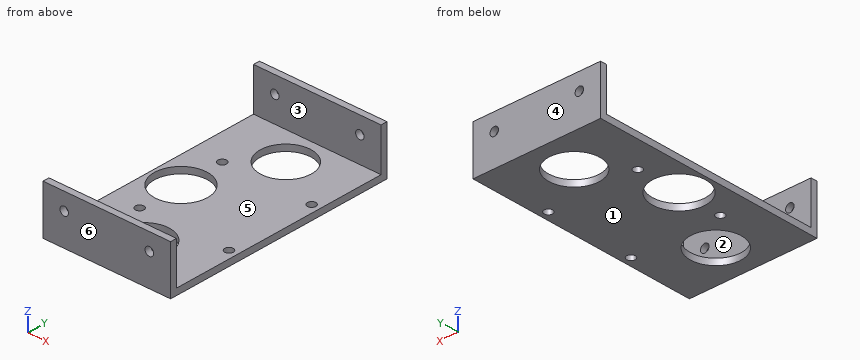
```python
from build123d import *

# Parameters (mm, degrees)
F0_W     = 30
F0_H     = 55
F0_R     = 1
F0_R_2   = 6
F0_R_3   = 6.25
F1_DEPTH = 1.5
F2_W     = 30
F2_H     = 1.5
F3_DEPTH = 10
F4_R     = 1
F5_DEPTH = 55.001


with BuildPart() as f1:
    # F0 (on Top) → F1 (new body)
    with BuildSketch(Plane.XY):
        with Locations((0, 7.5)):
            Rectangle(F0_W, F0_H)
        with Locations((-8, -3)):
            Circle(F0_R, mode=Mode.SUBTRACT)
        with Locations((0, -10.5)):
            Circle(F0_R_2, mode=Mode.SUBTRACT)
        with Locations((13, -3)):
            Circle(F0_R, mode=Mode.SUBTRACT)
        with Locations((-8, 7.5)):
            Circle(F0_R_3, mode=Mode.SUBTRACT)
        with Locations((-8, 18)):
            Circle(F0_R, mode=Mode.SUBTRACT)
        with Locations((13, 18)):
            Circle(F0_R, mode=Mode.SUBTRACT)
        with Locations((0, 25.5)):
            Circle(F0_R_2, mode=Mode.SUBTRACT)
    extrude(amount=F1_DEPTH)

    # F2 (on face) → F3 (join)
    with BuildSketch(Plane.XY.offset(1.5)):
        with Locations((0, 34.25)):
            Rectangle(F2_W, F2_H)
        with Locations((0, -19.25)):
            Rectangle(F2_W, F2_H)
    extrude(amount=F3_DEPTH)

    # F4 (on face) → F5 (cut, through all)
    with BuildSketch(Plane(origin=(0, 35, 0), x_dir=(-1, 0, 0), z_dir=(0, 1, 0))):
        with Locations((-10, 7.5)):
            Circle(F4_R)
        with Locations((10, 7.5)):
            Circle(F4_R)
    extrude(amount=-F5_DEPTH, mode=Mode.SUBTRACT)


solid = f1.part
```
Verification items for the finished model (mm, model axes). Face numbers are marked on the shaded views. A direction names the side the tool comes from. Round coordinates to 2 decimals unless told otherwise and drop trailing zeros. Write each loop counter-clockwise with the first axis right and the second up, starting at its lowest first coordinate (ties: lowest second). Pieces come first, ordered by that corner, then holes.
1. Section check A-A on x = 0. Enter the section's corners in (y, z).
2. Section check C-C on z = 5. Enter the section's corners in (x, y), plus the area to 3 significant figures.
3. Scan lines: L1, parallel to Y at x = 13, z = 0.6; L2, parallel to Y at x = -8, z = 0.45; L3, parallel to Y at x = -10.5, z = 9.25. Record each from-to range of solid material in increasing order.
4. Draft check along Y on the marked faces 1, 2, 3 and 4. Enter one of: +Y half, -Y half, draft (parallel to the pull), parting line (faces both ways), or undercut.
5. Section check D-D on z = 7.5. Enter the section's corners in (x, y), plus the area to 3 significant figures.
6. Gauge pin test, flat ends, axial feed: P1, Ø16, axis at x = -8, y = 7.5, coming from the +Z side; P2, Ø9.5, axis at x = 0, y = -10.5, coming from the +Z side. Record the tip position at first contact, or that the pin passes through.
7. Section check B-B on y = 18. Enter the section's corners in (x, z), plus the area to 3 significant figures.
8. Access from +Z, -Z, +X, -X, +Y, -Y to the whole of each face (thin tool, end or side, straight path). Record for the marked faces 5 and 6.
Answer:
1. outline: (-20, 0) - (-16.5, 0) - (-16.5, 1.5) - (-18.5, 1.5) - (-18.5, 11.5) - (-20, 11.5) - close; (-4.5, 0) - (19.5, 0) - (19.5, 1.5) - (-4.5, 1.5) - close; (31.5, 0) - (35, 0) - (35, 11.5) - (33.5, 11.5) - (33.5, 1.5) - (31.5, 1.5) - close
2. outline: (-15, -20) - (15, -20) - (15, -18.5) - (-15, -18.5) - close; (-15, 33.5) - (15, 33.5) - (15, 35) - (-15, 35) - close
2. area: 90.0 mm2
3. L1: y = -20 to -4, -2 to 17, 19 to 35
3. L2: y = -20 to -4, -2 to 1.25, 13.75 to 17, 19 to 35
3. L3: y = -20 to -18.5, 33.5 to 35
4. face 1: draft
4. face 2: undercut
4. face 3: undercut
4. face 4: +Y half
5. outline: (-15, -20) - (-11, -20) - (-11, -18.5) - (-15, -18.5) - close; (-15, 33.5) - (-11, 33.5) - (-11, 35) - (-15, 35) - close; (-9, -20) - (9, -20) - (9, -18.5) - (-9, -18.5) - close; (-9, 33.5) - (9, 33.5) - (9, 35) - (-9, 35) - close; (11, -20) - (15, -20) - (15, -18.5) - (11, -18.5) - close; (11, 33.5) - (15, 33.5) - (15, 35) - (11, 35) - close
5. area: 78.0 mm2
6. P1: stops at z = 1.5
6. P2: passes through
7. outline: (-15, 0) - (-9, 0) - (-9, 1.5) - (-15, 1.5) - close; (-7, 0) - (12, 0) - (12, 1.5) - (-7, 1.5) - close; (14, 0) - (15, 0) - (15, 1.5) - (14, 1.5) - close
7. area: 39.0 mm2
8. face 5: +Z, +X, -X
8. face 6: +Z, -Z, +X, -X, -Y
